The listing builds one solid part. Answer for the finished solid, in the listing's coordinates (mm). Give positions to 0.01 mm unless a question says otherwise; leave off trailing zeros. Write each loop counter-clockwise with the first axis right and the second up, starting at its lowest first coordinate (ties: lowest second). Pieces come first, ordered by that corner, then holes. Notation, with made-up numbers: (49.25, 72) - (59.25, 72) arc R5 cw to (59.25, 80) - close; hole circle Ø8 at (75.25, 75). An arc over 180 degrees is marked (long way). Answer in a Markdown table with one row per item. Add a question column.
from build123d import *

# Parameters (mm, degrees)
BOSS_EXTRUDE1_DEPTH = 10
SCALE2_SCALE        = 0.6
BOSS_EXTRUDE2_DEPTH = 430.08


with BuildPart() as part:
    # Sketch1 → Boss-Extrude1 (new body)
    with BuildSketch(Plane(origin=(0, 0, 0), x_dir=(1, 0, 0), z_dir=(0, 1, 0))):
        Polygon((219, 0), (219, 350.9), (98.6, 350.9), (0, 0), (0, -15), (98.6, -365.9), (219, -365.9), (219, -15), align=None)
    extrude(amount=BOSS_EXTRUDE1_DEPTH)


with BuildPart() as part_1:
    # Scale2: scaled about (131.165360429, 5, 7.5)
    add(part.part.scale(SCALE2_SCALE).moved(Location((52.466144172, 2, 3))))

    # Sketch2 → Boss-Extrude2 (add)
    with BuildSketch(Plane.XY.offset(222.54)):
        with BuildLine():
            Line((183.866144171, 8), (183.866144171, 2))
            ThreePointArc((183.866144171, 2), (184.617619122, 5), (183.866144171, 8))
        make_face()
    extrude(amount=-BOSS_EXTRUDE2_DEPTH)


solid = part_1.part
1. Section B-B (x = 92.5) is taken. Give the vertices of the cut face in (y, z), and give its area (3 significant figures).
2. Given pin 1 Ø3 at (y, z) = (7, -15.5) entering from -X, flat-ended and moving along its own axis, determine where the tip first touches the part or whether it passes through.
3. Section A-A (y = 5.05) is taken. Give the vertices of the cut face in (x, z).
4. Section C-C (z = 80) is taken. Give the vertices of the cut face in (x, y).
5. Straight lines are drawn through the part: L1, parallel to X at y = 3.1, z = -42.5; L2, parallel to X at y = 3.8, z = -179. For each, find the intervals that lie inside material, in ascending order. Write a range as [from, to].
Geometry check:
| question | item | result |
|---|---|---|
| 1 | outline | (2, -139.47) - (8, -139.47) - (8, 154.47) - (2, 154.47) - close |
| 1 | area | 1,760 mm² |
| 2 | pin 1 | x = 57.24 |
| 3 | outline | (52.47, 3) - (111.63, -207.54) - (184.62, -207.54) - (184.62, 222.54) - (111.63, 222.54) - (52.47, 12) - close |
| 4 | outline | (71.57, 2) - (183.87, 2) arc R6.36 ccw to (183.87, 8) - (71.57, 8) - close |
| 5 | L1 | [65.25, 184.33] |
| 5 | L2 | [103.61, 184.5] |
